```python
from build123d import *

# Parameters (mm, degrees)
SKETCH_1_W          = 49
SKETCH_1_H          = 21
SKETCH_1_R          = 4.1
SKETCH_1_R_2        = 1.6
EXTRUDE_1_DEPTH     = 57.8
SKETCH_4_W          = 98
SKETCH_4_H          = 11.45
CUT_EXTRUDE_3_DEPTH = 15.8
SKETCH_5_R          = 4.1
CUT_EXTRUDE_4_DEPTH = 42
SKETCH_6_W          = 98
SKETCH_6_H          = 21
EXTRUDE_2_DEPTH     = 2.5
SKETCH_7_R          = 1.6
SKETCH_7_R_2        = 1.534199572
CUT_EXTRUDE_5_DEPTH = 10
SKETCH_8_W          = 6
SKETCH_8_H          = 3
CUT_EXTRUDE_6_DEPTH = 7
FILLET_1_R          = 10
FILLET_2_R          = 10
FILLET_3_R          = 10
FILLET_4_R          = 10


with BuildPart() as part:
    # 草图1 → 凸台-拉伸1 (new body)
    # profile 1 of 6: a face of its own
    with BuildSketch(Plane.XY):
        with Locations((-24.5, 0)):
            Rectangle(SKETCH_1_W, SKETCH_1_H)
        with Locations((-40, -4.5)):
            Circle(SKETCH_1_R, mode=Mode.SUBTRACT)
        with Locations((-40, 7.5)):
            Circle(SKETCH_1_R_2, mode=Mode.SUBTRACT)
    # profile 2 of 6: a face of its own
    with BuildSketch(Plane.XY):
        with Locations((-40, -4.5)):
            Circle(SKETCH_1_R)
    # profile 3 of 6: a face of its own
    with BuildSketch(Plane.XY):
        with Locations((-40, 7.5)):
            Circle(SKETCH_1_R_2)
    # profile 4 of 6: a face of its own
    with BuildSketch(Plane.XY):
        with Locations((24.5, 0)):
            Rectangle(SKETCH_1_W, SKETCH_1_H)
        with Locations((40, -4.5)):
            Circle(SKETCH_1_R, mode=Mode.SUBTRACT)
        with Locations((40, 7.5)):
            Circle(SKETCH_1_R_2, mode=Mode.SUBTRACT)
    # profile 5 of 6: a face of its own
    with BuildSketch(Plane.XY):
        with Locations((40, -4.5)):
            Circle(SKETCH_1_R)
    # profile 6 of 6: a face of its own
    with BuildSketch(Plane.XY):
        with Locations((40, 7.5)):
            Circle(SKETCH_1_R_2)
    extrude(amount=EXTRUDE_1_DEPTH)

    # 草图4 → 切除-拉伸3 (cut)
    with BuildSketch(Plane(origin=(0, 0, 0), x_dir=(-1, 0, 0), z_dir=(0, 0, -1))):
        with Locations((0, -4.775)):
            Rectangle(SKETCH_4_W, SKETCH_4_H)
    extrude(amount=-CUT_EXTRUDE_3_DEPTH, mode=Mode.SUBTRACT)

    # 草图5 → 切除-拉伸4 (cut)
    with BuildSketch(Plane(origin=(0, 0, 15.8), x_dir=(-1, 0, 0), z_dir=(0, 0, -1))):
        with Locations((-40, -4.5)):
            Circle(SKETCH_5_R)
        with Locations((40, -4.5)):
            Circle(SKETCH_5_R)
    extrude(amount=-CUT_EXTRUDE_4_DEPTH, mode=Mode.SUBTRACT)

    # 草图6 → 凸台-拉伸2 (add)
    with BuildSketch(Plane.XY.offset(57.8)):
        Rectangle(SKETCH_6_W, SKETCH_6_H)
    extrude(amount=EXTRUDE_2_DEPTH)

    # 草图7 → 切除-拉伸5 (cut)
    with BuildSketch(Plane(origin=(0, 0, 0), x_dir=(-1, 0, 0), z_dir=(0, 0, -1))):
        with Locations((-40, 7.5)):
            Circle(SKETCH_7_R)
        with Locations((40, 7.5)):
            Circle(SKETCH_7_R_2)
    extrude(amount=-CUT_EXTRUDE_5_DEPTH, mode=Mode.SUBTRACT)

    # 草图8 → 切除-拉伸6 (cut)
    with BuildSketch(Plane(origin=(0, 10.5, 0), x_dir=(1, 0, 0), z_dir=(0, 1, 0))):
        with Locations((-40, -5)):
            Rectangle(SKETCH_8_W, SKETCH_8_H)
        with Locations((40, -5)):
            Rectangle(SKETCH_8_W, SKETCH_8_H)
    extrude(amount=-CUT_EXTRUDE_6_DEPTH, mode=Mode.SUBTRACT)

    # 圆角1
    # the kernel refuses this fillet: 10 mm, written as the material it takes off along each edge
    with BuildSketch(Plane(origin=(49, 10.5, -25), x_dir=(0, -1, 0), z_dir=(0, 0, 1))) as fillet_1_piece_1:
        with BuildLine():
            CenterArc((FILLET_1_R, -FILLET_1_R), FILLET_1_R, 90, 90)
            Line((0, -FILLET_1_R), (0, 0))
            Line((0, 0), (FILLET_1_R, 0))
        make_face()
    extrude(amount=110.3, mode=Mode.SUBTRACT)

    # 圆角2
    # the kernel refuses this fillet: 10 mm, written as the material it takes off along each edge
    with BuildSketch(Plane(origin=(-49, 10.5, 85.3), x_dir=(0, -1, 0), z_dir=(0, 0, -1))) as fillet_2_piece_1:
        with BuildLine():
            CenterArc((FILLET_2_R, -FILLET_2_R), FILLET_2_R, 90, 90)
            Line((0, -FILLET_2_R), (0, 0))
            Line((0, 0), (FILLET_2_R, 0))
        make_face()
    extrude(amount=110.3, mode=Mode.SUBTRACT)

    # 圆角3
    fillet_3_edges = [part.edges().sort_by_distance(p)[0] for p in [
        (-49, -10.5, 38.05),
    ]]
    fillet(fillet_3_edges, radius=FILLET_3_R)

    # 圆角4
    fillet_4_edges = [part.edges().sort_by_distance(p)[0] for p in [
        (49, -10.5, 38.05),
    ]]
    fillet(fillet_4_edges, radius=FILLET_4_R)


solid = part.part
```
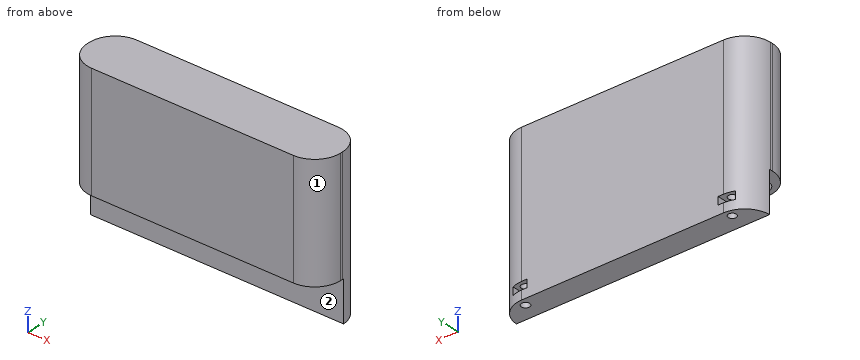
Here's how the part is built. I have some questions about the finished solid (model axes, mm). Face numbers are marked on the shaded views. A direction names the side the tool comes from. Coordinates: 2 decimals unless noted, no trailing zeros. Order: outer loops, then holes, each group sorted by start corner. A loop starts at its lowest first (then second) coordinate and runs counter-clockwise, first axis right, second up.
1) Imagine slicing it at B-B on x = -40. List the corners of the cut face in (y, z) for me, and give its area (3 significant figures).
2) I need wall thicknesses on line 1 (X direction, y = -1.5, z = 17); line 2 (Z direction, x = 6, y = -3); line 3 (Y direction, x = -40, z = 2.65). Which ranges of each line are inside material? Lowest first, please.
3) Which directions (+Z, -Z, +X, -X, +Y, -Y) give clear straight access to the entire face, cutting with the end or side of a thin tool? Please do the marked faces 1 and 2.
4) Imagine slicing it at D-D on y = -3.5. List the corners of the cut face in (x, z) for me, and give its area (3 significant figures).
5) Will these pins go through, and if not, where does the flat tip stop? pin 1 (6 mm diameter, centred on x = -21, z = 10.5, fed in from -Y); pin 2 (0.9 mm diameter, centred on x = 39, z = 5, fed in from +Y); pin 3 (3 mm diameter, centred on y = 8.5, z = 37, fed in from +X).
6) Imagine slicing it at A-A on z = 34. List the corners of the cut face in (x, y) for me.
7) Imagine slicing it at C-C on x = -29.5. List the corners of the cut face in (y, z) for me.
Response values:
1. outline: (-10.45, 15.8) - (-8.6, 15.8) - (-8.6, 57.8) - (-0.4, 57.8) - (-0.4, 15.8) - (0.95, 15.8) - (0.95, 0) - (5.97, 0) - (5.97, 3.5) - (3.5, 3.5) - (3.5, 6.5) - (5.97, 6.5) - (5.97, 10) - (9.03, 10) - (9.03, 6.5) - (10.45, 6.5) - (10.45, 60.3) - (-10.45, 60.3) - close; (9.03, 0) - (10.45, 0) - (10.45, 3.5) - (9.03, 3.5) - close
1. area: 693 mm2
2. line 1: x = -48.95 to -42.79, -37.21 to 37.21, 42.79 to 48.95
2. line 2: z = 15.8 to 60.3
2. line 3: y = 0.95 to 5.97, 9.03 to 10.45
3. face 1: +Z, -Z, +X, -Y
3. face 2: -Z, +X, -X, -Y
4. outline: (-48.54, 15.8) - (-43.98, 15.8) - (-43.98, 57.8) - (-36.02, 57.8) - (-36.02, 15.8) - (36.02, 15.8) - (36.02, 57.8) - (43.98, 57.8) - (43.98, 15.8) - (48.54, 15.8) - (48.54, 60.3) - (-48.54, 60.3) - close
4. area: 3,650 mm2
5. pin 1: stops at y = 0.95
5. pin 2: stops at y = 3.5
5. pin 3: stops at x = 46.6
6. outline: (-49, -0.5) arc R10 ccw to (-39, -10.5) - (39, -10.5) arc R10 ccw to (49, -0.5) - (49, 0.5) arc R10 ccw to (39, 10.5) - (-39, 10.5) arc R10 ccw to (-49, 0.5) - close; hole circle Ø8.2 at (-40, -4.5); hole circle Ø8.2 at (40, -4.5)
7. outline: (-10.5, 15.8) - (0.95, 15.8) - (0.95, 0) - (10.5, 0) - (10.5, 60.3) - (-10.5, 60.3) - close
